Geometry: see drawing. Coordinates: mm, zero at the bounding-box minimum. Coordinates: 2 decimals unless noted, no trailing zeros. Write each loop counter-clockwise with the first axis right and the second up, starting at its lowest first coordinate (ties: lowest second). Pieces come first, ordered by that corner, then holes.
1) Section query B-B (y = 40.5). Output: boundary loops of the cut face in (x, z), then the cut area to 3 significant figures.
2) Section query C-C (x = 58.42). Output: boundary loops of the cut face in (y, z), then the cut area to 3 significant figures.
3) Pin query (flat end, axial travel): pin 1 Ø4 at (y, z) = (40.5, 92.5) entering from -X; pin 2 Ø5.5 at (x, y) = (97.5, 40) entering from +Z; pin 3 Ø4 at (y, z) = (4.5, 92) entering from -X; pin 4 Ø5 at (x, y) = (49.5, 19) entering from -Z. Return the tip coordinate at first contact, or that it passes through.
4) Section query D-D (z = 159). Output: boundary loops of the cut face in (x, y), then the cut area to 3 significant figures.
5) Section query A-A (z = 99.5). Output: boundary loops of the cut face in (x, y), then the cut area to 3 significant figures.
6) Draft query along Y for the marked faces 1, 2 and 3. Return one class per face: pulls with the +Y half, pulls with the -Y half, needs draft (parallel to the pull), parting line crosses it, or undercut.
7) Line query: L1, parallel to Z at x = 52, y = 8; L2, parallel to X at y = 3.5, z = 48.5; L3, parallel to Z at x = 82, y = 39. Output: solid intervals per line, ascending.
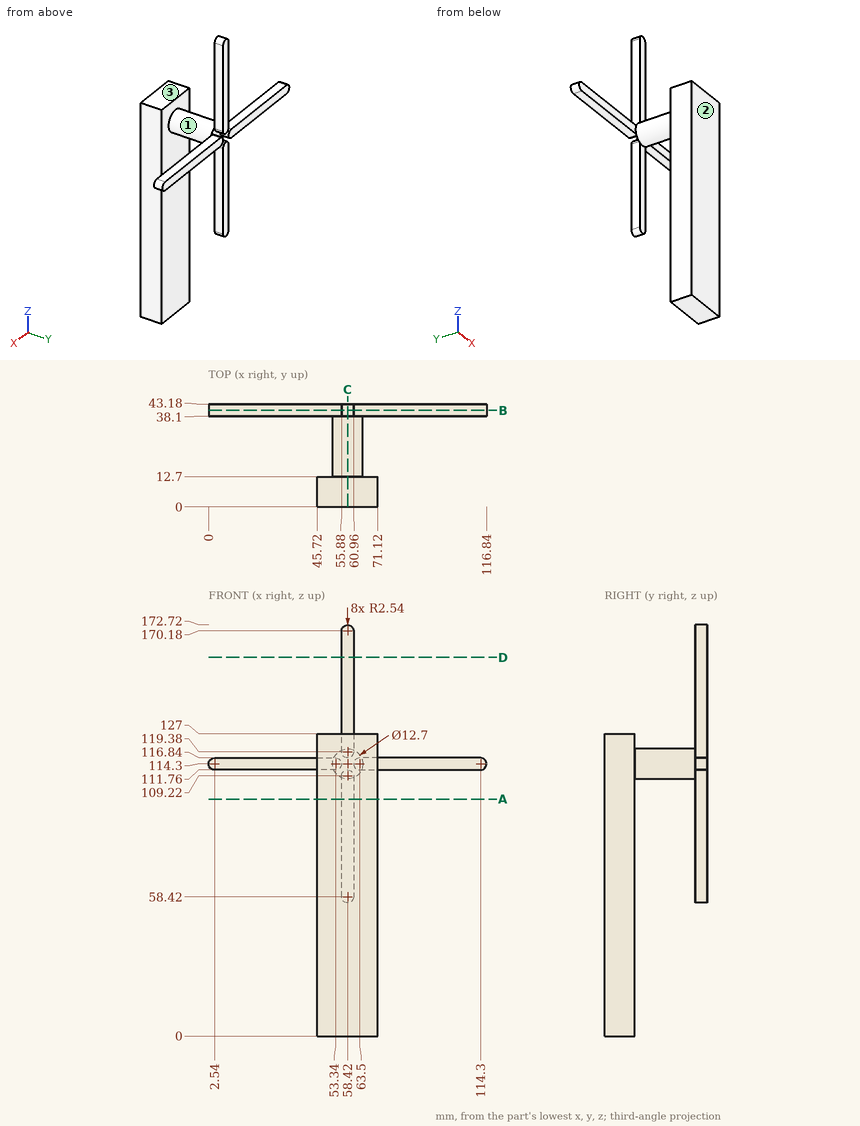
Answer:
1. outline: (2.54, 111.76) - (53.34, 111.76) arc R2.54 ccw to (53.34, 116.84) - (2.54, 116.84) arc R2.54 ccw to start; (55.88, 58.42) arc R2.54 ccw to (60.96, 58.42) - (60.96, 109.22) arc R2.54 ccw to (55.88, 109.22) - close; (55.88, 119.38) arc R2.54 ccw to (60.96, 119.38) - (60.96, 170.18) arc R2.54 ccw to (55.88, 170.18) - close; (63.5, 111.76) - (114.3, 111.76) arc R2.54 ccw to (114.3, 116.84) - (63.5, 116.84) arc R2.54 ccw to start
1. area: 1,110 mm2
2. outline: (0, 0) - (12.7, 0) - (12.7, 107.95) - (38.1, 107.95) - (38.1, 55.88) - (43.18, 55.88) - (43.18, 111.76) - (38.1, 111.76) - (38.1, 116.84) - (43.18, 116.84) - (43.18, 172.72) - (38.1, 172.72) - (38.1, 120.65) - (12.7, 120.65) - (12.7, 127) - (0, 127) - close
2. area: 2,500 mm2
3. pin 1: stops at x = 55.88
3. pin 2: stops at z = 116.84
3. pin 3: stops at x = 45.72
3. pin 4: passes through
4. outline: (55.88, 38.1) - (60.96, 38.1) - (60.96, 43.18) - (55.88, 43.18) - close
4. area: 25.8 mm2
5. outline: (45.72, 0) - (71.12, 0) - (71.12, 12.7) - (45.72, 12.7) - close; (55.88, 38.1) - (60.96, 38.1) - (60.96, 43.18) - (55.88, 43.18) - close
5. area: 348 mm2
6. face 1: undercut
6. face 2: pulls with the -Y half
6. face 3: needs draft
7. L1: z = 0 to 127
7. L2: x = 45.72 to 71.12
7. L3: z = 111.76 to 116.84
